Autodesk Fusion 360 part; units mm, degrees
sketch "Esquisse5" plane through (0, 0, 0) normal (0, 0, 1) x (1, 0, 0)
  line L0 (16.9, -17.9) -> (-16.9, -17.9)
  line L1 (-16.9, -17.9) -> (-16.9, 17.9)
  line L2 (-16.9, 17.9) -> (16.9, 17.9)
  line L3 (16.9, 17.9) -> (16.9, -17.9)
  line L4 (16.9, -17.9) -> (-16.9, 17.9) construction
  line L5 (-16.9, -17.9) -> (16.9, 17.9) construction
  circle A0 centre (-13.9, -14.9) radius 1.7
  line L6 (0, 0) -> (0, -17.9) construction
  line L7 (0, 0) -> (16.9, 0) construction
  circle A1 centre (13.9, -14.9) radius 1.7
  circle A2 centre (-13.9, 14.9) radius 1.7
  circle A3 centre (13.9, 14.9) radius 1.7
  line L8 (10.8, 9.17) -> (-10.8, 9.17)
  line L9 (-10.8, 9.17) -> (-10.8, -9.17)
  line L10 (-10.8, -9.17) -> (10.8, -9.17)
  line L11 (10.8, -9.17) -> (10.8, 9.17)
  line L12 (10.8, 9.17) -> (-10.8, -9.17) construction
  line L13 (-10.8, 9.17) -> (10.8, -9.17) construction
  line L14 (-10.05, -3.25) -> (10.05, -3.25)
  line L15 (10.05, -3.25) -> (10.05, 3.25)
  line L16 (10.05, 3.25) -> (-10.05, 3.25)
  line L17 (-10.05, 3.25) -> (-10.05, -3.25)
  line L18 (-10.05, -3.25) -> (10.05, 3.25) construction
  line L19 (10.05, -3.25) -> (-10.05, 3.25) construction
  dimension "d54" = 33.8
  dimension "d55" = 35.8
  dimension "d56" = 3.4
  dimension "d57" = 3
  dimension "d58" = 3
  dimension "d59" = 21.6
  dimension "d60" = 18.34
  dimension "d61" = 20.1
  dimension "d62" = 6.5
extrude "Extrusion3" add sketch "Esquisse5" against normal blind 3 contours L8 L9 L10 L11
extrude "Extrusion4" add sketch "Esquisse5" along normal blind 2 contours L0 L1 L2 L3
extrude "Extrusion5" add sketch "Esquisse5" along normal blind 7 contours L8 L9 L10 L11
sketch "Esquisse6" plane through (0, 9.17, 0) normal (0, 1, 0) x (-1, 0, 0)
  line L0 (-10.8, 2) -> (10.8, 2)
  line L1 (10.8, 2) -> (10.8, 7)
  line L2 (10.8, 7) -> (-10.8, 7)
  line L3 (-10.8, 7) -> (-10.8, 2)
  circle A0 centre (4.75, 3.75) radius 1.25
  circle A1 centre (-4.75, 3.75) radius 1.25
  line L4 (0, 2) -> (0, 7) construction
  dimension "d69" = 2.5
  dimension "d70" = 2.5
  dimension "d71" = 3.25
  dimension "d72" = 3.25
  dimension "d73" = 9.5
extrude "Extrusion6" cut sketch "Esquisse6" against normal through all contours A0 | A1
sketch "Esquisse7" plane through (0, 0, 7) normal (0, 0, 1) x (-1, 0, 0)
  line L0 (10.05, 3.25) -> (10.05, -3.25)
  line L1 (10.05, -3.25) -> (-10.05, -3.25)
  line L2 (-10.05, -3.25) -> (-10.05, 3.25)
  line L3 (-10.05, 3.25) -> (10.05, 3.25)
  line L4 (-10.8, 9.17) -> (-10.8, -9.17)
  line L5 (-10.8, -9.17) -> (10.8, -9.17)
  line L6 (10.8, -9.17) -> (10.8, 9.17)
  line L7 (10.8, 9.17) -> (-10.8, 9.17)
  line L8 (10.8, -6.25) -> (-10.8, -6.25)
  line L9 (-10.05, -3.25) -> (10.05, -3.25)
  line L10 (10.8, 6.25) -> (-10.8, 6.25)
  dimension "d76" = 3
  dimension "d77" = 3
extrude "Extrusion7" cut sketch "Esquisse7" against normal blind 5 contours L4 L6 L7 L10 | L4 L5 L6 L8
move_face "DécalerLesFaces1" offset 1 1 faces at (10.8, -2.0833, 3.6667)
move_face "DécalerLesFaces2" offset 1 1 faces at (-10.8, 2.0833, 3.6667)
equation "d70 = d69"
equation "d71 = 2 mm + ( 2.5 / 2 ) * 1 mm"
equation "d72 = d71"
equation "d73 = 7 mm + d69"
Work out the finished part from the listing and answer in its coordinate system (mm). A direction names the side the tool comes from. Coordinates: 2 decimals unless noted, no trailing zeros. Loops run counter-clockwise (first coordinate to the right, second up) from the corner with the lowest first, then second, coordinate; pieces in that order, holes last. Notation, with made-up numbers: M 7.5,55.25 L 19.5,55.25 A16 cw 19.5,59.25 Z; hole C 86,10 d10. An arc over 180 degrees is marked long. Answer in a Markdown table with one row per item. Add a question column.
1. A tool of negligible diameter and unlimited length cuts with its end or side. For faces 4 (the flat face through (0, 3.25, 2)), 5 (the flat face through (-11.8, 0, 4)), 6 (the flat face through (10.8, 0, -1)), 7 (the flat face through (0, 9.17, -1)), from which of +Z, -Z, +X, -X, +Y, -Y can it reach the whole face along a straight path? Write none if from no direction.
2. The mould has two halves that part along Z. Classify faces 1 (the flat face through (0, 4, 7)), 2 (the cylindrical face through (5.02, -4.73, 2.53)), 3 (the cylindrical face through (12.65, -16.05, 0.99)): pulls with the +Z half, pulls with the -Z half, needs draft (parallel to the pull), parting line crosses it, or undercut.
3. Find section A-A, the plane y = -14.9. Write down the section's boundary in (x, z).
4. Flat-ended cylindrical pins translate along their axes: P1, Ø3, axis at x = -4.75, z = 3.75, coming from the -Y side; P2, Ø0.9, axis at y = 3.5, z = -2, coming from the +X side; P3, Ø5.5, axis at x = 13.9, y = -14.9, coming from the +Z side; P4, Ø2, axis at x = 4.75, z = 3.75, coming from the +Y side. Find the tip coordinate at first contact, or state that the pin passes through.
5. Find section C-C, the plane x = -1.5. Write down the section's boundary in (y, z).
6. Find section B-B, the plane z = 5.75. Write down the section's boundary in (x, y), then the cut area to 3 significant figures.
7. Consider L1, parallel to Y at x = 13.9, z = 1.5; L2, parallel to X at y = -14.9, z = 0.95; L3, parallel to Y at x = 9, z = 6.75. Determine where each line is inside the solid, lowest interval first.
8. Find section D-D, the plane z = 1.5. Write down the section's boundary in (x, y), then the cut area to 3 significant figures.
Reported:
| question | item | result |
|---|---|---|
| 1 | face 4 | +Z, -Z |
| 1 | face 5 | +Z, -X, +Y, -Y |
| 1 | face 6 | -Z, +X, +Y, -Y |
| 1 | face 7 | -Z, +X, -X, +Y |
| 2 | face 1 | pulls with the +Z half |
| 2 | face 2 | undercut |
| 2 | face 3 | needs draft |
| 3 | outline | M -16.9,0 L -15.6,0 L -15.6,2 L -16.9,2 Z; M -12.2,0 L 12.2,0 L 12.2,2 L -12.2,2 Z; M 15.6,0 L 16.9,0 L 16.9,2 L 15.6,2 Z |
| 4 | P1 | stops at y = -6.25 |
| 4 | P2 | stops at x = 10.8 |
| 4 | P3 | stops at z = 2 |
| 4 | P4 | passes through |
| 5 | outline | M -17.9,0 L -9.17,0 L -9.17,-3 L -3.25,-3 L -3.25,7 L -6.25,7 L -6.25,2 L -17.9,2 Z; M 3.25,-3 L 9.17,-3 L 9.17,0 L 17.9,0 L 17.9,2 L 6.25,2 L 6.25,7 L 3.25,7 Z |
| 6 | outline | M -11.8,-6.25 L 11.8,-6.25 L 11.8,6.25 L -11.8,6.25 Z; hole M -10.05,-3.25 L 10.05,-3.25 L 10.05,3.25 L -10.05,3.25 Z |
| 6 | area | 164 mm^2 |
| 7 | L1 | y = -17.9 to -16.6, -13.2 to 13.2, 16.6 to 17.9 |
| 7 | L2 | x = -16.9 to -15.6, -12.2 to 12.2, 15.6 to 16.9 |
| 7 | L3 | y = -6.25 to -3.25, 3.25 to 6.25 |
| 8 | outline | M -16.9,-17.9 L 16.9,-17.9 L 16.9,17.9 L -16.9,17.9 Z; hole C -13.9,-14.9 d3.4; hole C -13.9,14.9 d3.4; hole M -10.05,-3.25 L 10.05,-3.25 L 10.05,3.25 L -10.05,3.25 Z; hole C 13.9,-14.9 d3.4; hole C 13.9,14.9 d3.4 |
| 8 | area | 1,040 mm^2 |
